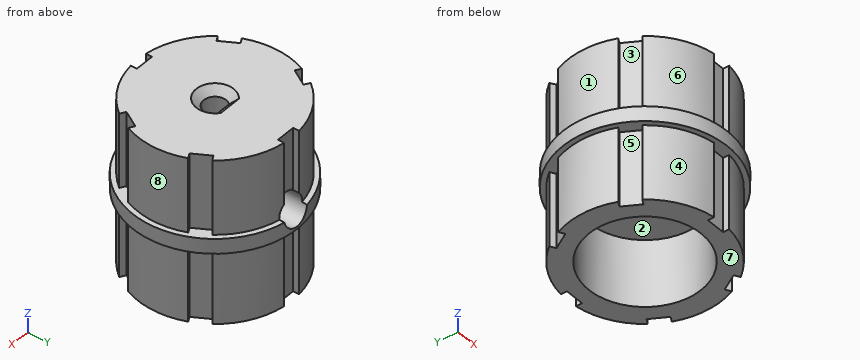
```python
from build123d import *

# Parameters (mm, degrees)
EXTRUDE_1_DEPTH          = 22
SKETCH_2_R               = 7.5
CUT_EXTRUDE_1_DEPTH      = 9
CUT_EXTRUDE_3_DEPTH      = 1
CUT_EXTRUDE_3_DEPTH_BACK = 8.42975
SKETCH_4_R               = 1.9
CHAMFER_1_SIZE           = 1
EXTRUDE_START            = -10
SKETCH_5_R               = 11
SKETCH_5_R_2             = 9.429749991
EXTRUDE_2_DEPTH          = 2
CUT_EXTRUDE_4_DEPTH      = 2
CUT_EXTRUDE_4_DEPTH_BACK = 2
SKETCH_6_R               = 1.9


with BuildPart() as part:
    # Эскиз1 → Бобышка-Вытянуть1 (new body)
    with BuildSketch(Plane.XY):
        with BuildLine():
            Line((13.201310027, -7.85542296), (13.90326512, -8.260696921))
            ThreePointArc((13.90326512, -8.260696921), (14.718656981, -4.240400213), (13.903265122, -0.220103504))
            Line((13.903265122, -0.220103504), (13.201310027, -0.625377467))
            Line((13.201310027, -0.625377467), (11.931310033, 1.574327047))
            Line((11.931310033, 1.574327047), (12.633265127, 1.979601009))
            ThreePointArc((12.633265127, 1.979601009), (9.559281984, 4.695899416), (5.669906988, 5.999897702))
            Line((5.669906988, 5.999897702), (5.669906988, 5.189349779))
            Line((5.669906988, 5.189349779), (3.129906988, 5.189349779))
            Line((3.129906988, 5.189349779), (3.129906988, 5.999897708))
            ThreePointArc((3.129906988, 5.999897708), (-0.759468012, 4.69589942), (-3.833451156, 1.979601011))
            Line((-3.833451156, 1.979601011), (-3.131496059, 1.574327046))
            Line((-3.131496059, 1.574327046), (-4.401496055, -0.625377472))
            Line((-4.401496055, -0.625377472), (-5.103451147, -0.22010351))
            ThreePointArc((-5.103451147, -0.22010351), (-5.918843009, -4.240400218), (-5.10345115, -8.260696926))
            Line((-5.10345115, -8.260696926), (-4.401496056, -7.855422963))
            Line((-4.401496056, -7.855422963), (-3.13149606, -10.055127481))
            Line((-3.13149606, -10.055127481), (-3.833451154, -10.460401444))
            ThreePointArc((-3.833451154, -10.460401444), (-0.759468012, -13.17669985), (3.129906983, -14.480698136))
            Line((3.129906983, -14.480698136), (3.129906983, -13.670150213))
            Line((3.129906983, -13.670150213), (5.669906983, -13.670150213))
            Line((5.669906983, -13.670150213), (5.669906983, -14.480698142))
            ThreePointArc((5.669906983, -14.480698142), (9.559281984, -13.176699854), (12.633265129, -10.460401443))
            Line((12.633265129, -10.460401443), (11.931310031, -10.055127478))
            Line((11.931310031, -10.055127478), (13.201310027, -7.85542296))
        make_face()
        with BuildLine():
            Line((3.281873001, -3.240400222), (5.517940979, -3.240400222))
            ThreePointArc((5.517940979, -3.240400222), (4.39990699, -5.740400222), (3.281873001, -3.240400222))
        make_face(mode=Mode.SUBTRACT)
    extrude(amount=EXTRUDE_1_DEPTH)

    # Эскиз2 → Вырез-Вытянуть1 (cut)
    with BuildSketch(Plane(origin=(0, 0, 0), x_dir=(-1, 0, 0), z_dir=(0, 0, -1))):
        with Locations((-4.39990699, -4.240400222)):
            Circle(SKETCH_2_R)
    extrude(amount=-CUT_EXTRUDE_1_DEPTH, mode=Mode.SUBTRACT)

    # Эскиз4 → Вырез-Вытянуть3 (cut, two sides: drawn at the far end of the back side and taken through both)
    with BuildSketch(Plane(origin=(0, 5.189349779, 0), x_dir=(1, 0, 0), z_dir=(0, 1, 0)).offset(-CUT_EXTRUDE_3_DEPTH_BACK)):
        with Locations(Location((4.428692677, -12.248697559, 0), (0, 0, 55.020131728))):
            Circle(SKETCH_4_R)
    extrude(amount=CUT_EXTRUDE_3_DEPTH + CUT_EXTRUDE_3_DEPTH_BACK, mode=Mode.SUBTRACT)

    # Фаска1
    chamfer_1_edges = [part.edges().sort_by_distance(p)[0] for p in [
        (4.39990699, -5.740400222, 22),
        (4.39990699, -3.240400222, 22),
        (4.39990699, -3.240400222, 9),
        (4.39990699, -5.740400222, 9),
    ]]
    chamfer(chamfer_1_edges, length=CHAMFER_1_SIZE)

    # Эскиз5 → Бобышка-Вытянуть2 (add)
    with BuildSketch(Plane(origin=(0, 0, 0), x_dir=(-1, 0, 0), z_dir=(0, 0, -1)).offset(EXTRUDE_START)):
        with Locations((-4.39990699, -4.240400222)):
            Circle(SKETCH_5_R)
        with Locations((-4.39990699, -4.240400222)):
            Circle(SKETCH_5_R_2, mode=Mode.SUBTRACT)
    extrude(amount=-EXTRUDE_2_DEPTH)

    # Эскиз6 → Вырез-Вытянуть4 (cut, two sides: drawn at the far end of the back side and taken through both)
    with BuildSketch(Plane(origin=(0, 5.189349779, 0), x_dir=(1, 0, 0), z_dir=(0, 1, 0)).offset(-CUT_EXTRUDE_4_DEPTH_BACK)):
        with Locations(Location((4.428692677, -12.248697559, 0), (0, 0, 55.020131728))):
            Circle(SKETCH_6_R)
    extrude(amount=CUT_EXTRUDE_4_DEPTH + CUT_EXTRUDE_4_DEPTH_BACK, mode=Mode.SUBTRACT)


solid = part.part
```
Could you check a few things on this model? Use its own coordinates, in mm. Face numbers are marked on the shaded views. A direction names the side the tool comes from. Coordinates: 2 decimals unless noted, no trailing zeros. Write each loop counter-clockwise with the first axis right and the second up, starting at its lowest first coordinate (ties: lowest second). Pieces come first, ordered by that corner, then holes. Notation, with made-up numbers: (78.5, -29.5) - (85.5, -29.5) arc R18 ccw to (85.5, 3.5) - close; hole circle Ø10 at (26, -36.5). An arc over 180 degrees is marked (long way). Use a Markdown table: item, result.
Q1. Imagine slicing it at A-A (z = 17.5). List the corners of the cut face in (x, y) for me, and give its area (3 significant figures).
Geometry check:
| item | result |
|---|---|
| outline | (-5.1, -8.26) - (-4.4, -7.86) - (-3.13, -10.06) - (-3.83, -10.46) arc R10.32 ccw to (3.13, -14.48) - (3.13, -13.67) - (5.67, -13.67) - (5.67, -14.48) arc R10.32 ccw to (12.63, -10.46) - (11.93, -10.06) - (13.2, -7.86) - (13.9, -8.26) arc R10.32 ccw to (13.9, -0.22) - (13.2, -0.63) - (11.93, 1.57) - (12.63, 1.98) arc R10.32 ccw to (5.67, 6) - (5.67, 5.19) - (3.13, 5.19) - (3.13, 6) arc R10.32 ccw to (-3.83, 1.98) - (-3.13, 1.57) - (-4.4, -0.63) - (-5.1, -0.22) arc R10.32 ccw to start; hole (3.28, -3.24) arc R1.5 ccw (long way) to (5.52, -3.24) - close |
| area | 315 mm2 |
Q2. Imagine slicing it at D-D (z = 12.75). List the corners of the cut face in (x, y) for me.
Geometry check:
| item | result |
|---|---|
| outline | (-5.1, -8.26) - (-4.4, -7.86) - (-3.13, -10.06) - (-3.83, -10.46) arc R10.32 ccw to (3.13, -14.48) - (3.13, -13.67) - (5.67, -13.67) - (5.67, -14.48) arc R10.32 ccw to (12.63, -10.46) - (11.93, -10.06) - (13.2, -7.86) - (13.9, -8.26) arc R10.32 ccw to (13.9, -0.22) - (13.2, -0.63) - (11.93, 1.57) - (12.63, 1.98) arc R10.32 ccw to (6.26, 5.91) - (6.26, -3.24) - (5.52, -3.24) arc R1.5 cw (long way) to (3.28, -3.24) - (2.6, -3.24) - (2.6, 5.92) arc R10.32 ccw to (-3.83, 1.98) - (-3.13, 1.57) - (-4.4, -0.63) - (-5.1, -0.22) arc R10.32 ccw to start |
Q3. Which directions (+Z, -Z, +X, -X, +Y, -Y) give clear straight access to the entire face, cutting with the end or side of a thin tool? Please do the marked faces 1, 2, 3 and 4.
Geometry check:
| item | result |
|---|---|
| face 1 | +Z, -X |
| face 2 | -Z |
| face 3 | +Z |
| face 4 | -Z, -X, -Y |
Q4. Thinking about a two-plate mould opening in X: for the marked faces 5, 6, 7 and 8, which applies, +X half, -X half, draft (parallel to the pull), parting line (faces both ways), or undercut?
Geometry check:
| item | result |
|---|---|
| face 5 | undercut |
| face 6 | -X half |
| face 7 | draft |
| face 8 | +X half |
Q5. Please list where these lines run through material, in increasing order: L1, parallel to Y at x = 4.25, z = 1.25; L2, parallel to Z at x = 6.5, y = -0.25; L3, parallel to X at y = 1.25, z = 6.
Geometry check:
| item | result |
|---|---|
| L1 | y = -13.67 to -11.74, 3.26 to 5.19 |
| L2 | z = 9 to 22 |
| L3 | x = -3.32 to -0.71, 9.51 to 12.12 |
Q6. I'm going to push flat-ended pins straight in: pin 1 Ø3 at (x, z) = (4, 4) entering from -Y; pin 2 Ø0.6 at (y, z) = (-14, 5.5) entering from +X; pin 3 Ø1.5 at (y, z) = (3, 12.5) entering from +X; pin 4 Ø12 at (x, y) = (3.5, 4) entering from -Z. Where does each tip first touch, or does it pass through?
Geometry check:
| item | result |
|---|---|
| pin 1 | stops at y = -14.48 |
| pin 2 | stops at x = 8.52 |
| pin 3 | stops at x = 13.14 |
| pin 4 | stops at z = 0 |
Q7. Imagine slicing it at C-C (x = 10.5). List the corners of the cut face in (y, z) for me, and give its area (3 significant figures).
Geometry check:
| item | result |
|---|---|
| outline | (-13.39, 10) - (-12.56, 10) - (-12.56, 0) - (-8.6, 0) - (-8.6, 9) - (0.12, 9) - (0.12, 0) - (4.08, 0) - (4.08, 10) - (4.91, 10) - (4.91, 12) - (4.08, 12) - (4.08, 22) - (-12.56, 22) - (-12.56, 12) - (-13.39, 12) - close |
| area | 291 mm2 |
Q8. Imagine slicing it at B-B (y = -1). List the corners of the cut face in (x, z) for me.
Geometry check:
| item | result |
|---|---|
| outline | (-6.11, 10) - (-5.4, 10) - (-5.4, 0) - (-2.36, 0) - (-2.36, 9) - (11.16, 9) - (11.16, 0) - (14.2, 0) - (14.2, 10) - (14.91, 10) - (14.91, 12) - (14.2, 12) - (14.2, 22) - (-5.4, 22) - (-5.4, 12) - (-6.11, 12) - close; hole circle Ø3.8 at (4.43, 12.25) |
